Source: CAD feature listing. Evaluate the final solid. Frame: model axes, mm. Face numbers are marked on the shaded views. A direction names the side the tool comes from. Round coordinates to 2 decimals unless told otherwise and drop trailing zeros. Loops run counter-clockwise (first coordinate to the right, second up) from the corner with the lowest first, then second, coordinate; pieces in that order, holes last. Notation, with made-up numbers: M 35.5,48 L 79.5,48 A10 ccw 79.5,58 Z; hole C 56,35.25 d10. An arc over 180 degrees is marked long. Write each question's results on one line, items separated by ' | '. Start each with the question number.
1. Contact query for flat-ended pins moving along their axis: pin 1 Ø1.5 at (y, z) = (3.5, 37) entering from -X; pin 2 Ø2 at (y, z) = (2.5, 15) entering from -X; pin 3 Ø1.5 at (y, z) = (3.5, 53) entering from +X. Output: stop coordinate, or through.
2. Set-up query: the marked faces 4 and 5. Return all of +Z, -Z, +X, -X, +Y, -Y with unobstructed straight access to the full face (end or side cutting, diameter ignored); none if empty.
3. Section A-A on x = 11.8. Output: boundary loops of the cut face in (y, z), and give its area (3 significant figures).
4. Ray query, line 1 (Z direction, x = 0, y = 3.35); line 2 (X direction, y = 3.35, z = 0); line 3 (Z direction, x = 4.5, y = 1.3). Return the intervals inside material, ascending.
5. Draft query along Y for the marked faces 1, 2 and 3. Return one class per face: released by +Y, released by -Y, zero draft, split by the parting line, or undercut.
6. Section B-B on z = 0. Output: boundary loops of the cut face in (x, y).
7. Section D-D on z = 44.5. Output: boundary loops of the cut face in (x, y), and give its area (3 significant figures).
8. Section C-C on y = 4.1. Give the number of separate pieces and of enclosed holes in the cut face, and give its area (3 significant figures).
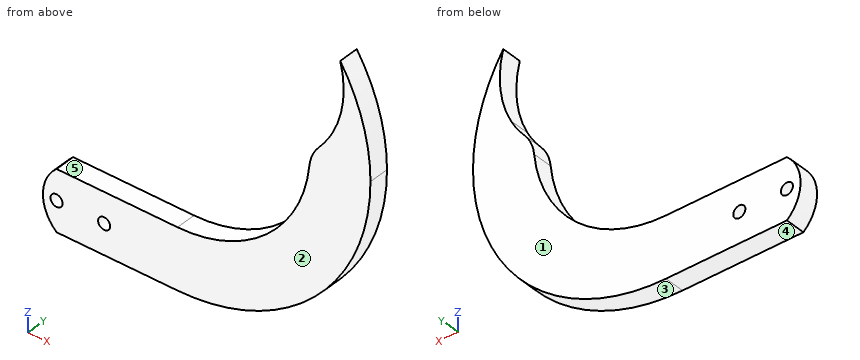
from build123d import *

# Parameters (mm, degrees)
SKETCH1_R           = 1.5
BOSS_EXTRUDE1_DEPTH = 5
CUT_EXTRUDE1_DEPTH  = 10
BOSS_EXTRUDE2_DEPTH = 5
CUT_EXTRUDE2_DEPTH  = 10
FILLET1_R           = 10


with BuildPart() as part:
    # Sketch1 → Boss-Extrude1 (new body)
    with BuildSketch(Plane(origin=(0, 0, 0), x_dir=(1, 0, 0), z_dir=(0, 1, 0))):
        with BuildLine():
            ThreePointArc((30, 7.5), (22.5, 0), (30, -7.5))
            Line((30, -7.5), (0, -7.5))
            ThreePointArc((0, -7.5), (-7.5, 0), (0, 7.5))
            Line((0, 7.5), (30, 7.5))
        make_face()
        with Locations((11.8, 0)):
            Circle(SKETCH1_R, mode=Mode.SUBTRACT)
        Circle(SKETCH1_R, mode=Mode.SUBTRACT)
        with BuildLine():
            ThreePointArc((30, -7.5), (37.5, 0), (30, 7.5))
            ThreePointArc((30, 7.5), (22.5, 0), (30, -7.5))
        make_face()
        with BuildLine():
            ThreePointArc((62.875, -40.375), (53.246135432, -17.128864568), (30, -7.5))
            ThreePointArc((30, -7.5), (37.5, 0), (30, 7.5))
            ThreePointArc((30, 7.5), (63.852737149, -6.522262851), (77.875, -40.375))
            ThreePointArc((77.875, -40.375), (70.375, -47.875), (62.875, -40.375))
        make_face()
    extrude(amount=BOSS_EXTRUDE1_DEPTH)

    # Sketch2 → Cut-Extrude1 (cut)
    with BuildSketch(Plane(origin=(0, 5, 0), x_dir=(1, 0, 0), z_dir=(0, 1, 0))):
        with BuildLine():
            ThreePointArc((0, 7.5), (-7.5, 0), (0, -7.5))
            ThreePointArc((0, -7.5), (-3.385621722, 0), (0, 7.5))
        make_face()
    extrude(amount=-CUT_EXTRUDE1_DEPTH, mode=Mode.SUBTRACT)

    # Sketch3 → Boss-Extrude2 (add)
    with BuildSketch(Plane(origin=(0, 5, 0), x_dir=(1, 0, 0), z_dir=(0, 1, 0))):
        with BuildLine():
            ThreePointArc((77.875, -40.375), (74.960699845, -46.309758372), (68.482638152, -47.632338812))
            ThreePointArc((68.482638152, -47.632338812), (71.093194767, -56.399789932), (70.375, -65.519406222))
            ThreePointArc((70.375, -65.519406222), (75.960053745, -53.494557579), (77.875, -40.375))
        make_face()
    extrude(amount=-BOSS_EXTRUDE2_DEPTH)

    # Sketch4 → Cut-Extrude2 (cut)
    with BuildSketch(Plane(origin=(0, 5, 0), x_dir=(1, 0, 0), z_dir=(0, 1, 0))):
        with BuildLine():
            ThreePointArc((62.875, -40.375), (64.440241628, -44.960699845), (68.482638152, -47.632338812))
            ThreePointArc((68.482638152, -47.632338812), (66.014466289, -43.744319779), (62.875, -40.375))
        make_face()
    extrude(amount=-CUT_EXTRUDE2_DEPTH, mode=Mode.SUBTRACT)

    # Fillet1
    fillet1_edges = [part.edges().sort_by_distance(p)[0] for p in [
        (62.875, 2.5, 40.375),
    ]]
    fillet(fillet1_edges, radius=FILLET1_R)


solid = part.part
Taken from the geometry:
1) pin 1: x = 62.62 | pin 2: x = 49.62 | pin 3: x = 76.31
2) face 4: -Z, +X, -X, +Y, -Y | face 5: +Z, -X, +Y, -Y
3) outline: M 0,-7.5 L 5,-7.5 L 5,-1.5 L 0,-1.5 Z; M 0,1.5 L 5,1.5 L 5,7.5 L 0,7.5 Z | area: 60.0 mm^2
4) line 1: -7.5 to -1.5, 1.5 to 7.5 | line 2: -3.39 to -1.5, 1.5 to 10.3, 13.3 to 55.73 | line 3: -7.5 to 7.5
5) face 1: released by +Y | face 2: released by -Y | face 3: zero draft
6) outline: M -3.39,0 L -1.5,0 L -1.5,5 L -3.39,5 Z; M 1.5,0 L 10.3,0 L 10.3,5 L 1.5,5 Z; M 13.3,0 L 55.73,0 L 55.73,5 L 13.3,5 Z
7) outline: M 66.58,0 L 77.69,0 L 77.69,5 L 66.58,5 Z | area: 55.6 mm^2
8) separate pieces: 1 | enclosed holes: 2 | area: 1,580 mm^2
